from build123d import *

# Parameters (mm, degrees)
F1_DEPTH = 612.95
F3_DEPTH = 127.001


with BuildPart() as f1:
    # F0 (on Front) → F1 (new body)
    with BuildSketch(Plane.XZ):
        with BuildLine():
            Line((-53.95, -63.5), (53.95, -63.5))
            ThreePointArc((53.95, -63.5), (60.70287, -60.70287), (63.5, -53.95))
            Line((63.5, -53.95), (63.5, 53.95))
            ThreePointArc((63.5, 53.95), (60.70287, 60.70287), (53.95, 63.5))
            Line((53.95, 63.5), (-53.95, 63.5))
            ThreePointArc((-53.95, 63.5), (-60.70287, 60.70287), (-63.5, 53.95))
            Line((-63.5, 53.95), (-63.5, -53.95))
            ThreePointArc((-63.5, -53.95), (-60.70287, -60.70287), (-53.95, -63.5))
        make_face()
        with BuildLine():
            ThreePointArc((58.7255, -53.9505), (57.326935, -57.326935), (53.9505, -58.7255))
            Line((53.9505, -58.7255), (-53.9505, -58.7255))
            ThreePointArc((-53.9505, -58.7255), (-57.326935, -57.326935), (-58.7255, -53.9505))
            Line((-58.7255, -53.9505), (-58.7255, 53.9505))
            ThreePointArc((-58.7255, 53.9505), (-57.326935, 57.326935), (-53.9505, 58.7255))
            Line((-53.9505, 58.7255), (53.9505, 58.7255))
            ThreePointArc((53.9505, 58.7255), (57.326935, 57.326935), (58.7255, 53.9505))
            Line((58.7255, 53.9505), (58.7255, -53.9505))
        make_face(mode=Mode.SUBTRACT)
    extrude(amount=F1_DEPTH)

    # F2 (on face) → F3 (cut, through all)
    with BuildSketch(Plane.XY.offset(63.5)):
        with BuildLine():
            Line((-31.75, -142.1), (31.75, -142.1))
            ThreePointArc((31.75, -142.1), (36.240128, -140.240128), (38.1, -135.75))
            Line((38.1, -135.75), (38.1, -110.35))
            ThreePointArc((38.1, -110.35), (36.240128, -105.859872), (31.75, -104))
            Line((31.75, -104), (-31.75, -104))
            ThreePointArc((-31.75, -104), (-36.240128, -105.859872), (-38.1, -110.35))
            Line((-38.1, -110.35), (-38.1, -135.75))
            ThreePointArc((-38.1, -135.75), (-36.240128, -140.240128), (-31.75, -142.1))
        make_face()
    extrude(amount=-F3_DEPTH, mode=Mode.SUBTRACT)


solid = f1.part
Source: CAD feature listing. Evaluate the final solid. Frame: model axes, mm. A direction names the side the tool comes from. Coordinates: 2 decimals unless noted, no trailing zeros. Loops run counter-clockwise (first coordinate to the right, second up) from the corner with the lowest first, then second, coordinate; pieces in that order, holes last. Notation, with made-up numbers: M 14,-33.75 L 37,-33.75 A28 ccw 37,-6.75 Z; hole C -16,-6.5 d8. An arc over 180 degrees is marked long. Answer in a Markdown table with one row per item.
Q1. First-contact query: pin 1 (2.5 mm diameter, centred on y = -123.5, z = 60.5, fed in from -X); pin 2 (4 mm diameter, centred on y = -121.5, z = 62, fed in from +X); pin 3 (4 mm diameter, centred on y = -120.5, z = -60, fed in from -X). Flat tips, straight axial feed; report the tip coordinate or a pass-through.
Answers below:
| item | result |
|---|---|
| pin 1 | stops at x = -61.89 |
| pin 2 | stops at x = 61.34 |
| pin 3 | stops at x = -62.6 |
Q2. Draft query along Z for faces 3 (the flat face through (-1, -302, -63.5)), 4 (the flat face through (1, -302, 63.5)), 5 (the flat face through (58.726, -302, 1)), 6 (the flat face through (-63.5, -302, 1)). Return one class per face: pulls with the +Z half, pulls with the -Z half, needs draft (parallel to the pull), parting line crosses it, or undercut.
Answers below:
| item | result |
|---|---|
| face 3 | pulls with the -Z half |
| face 4 | pulls with the +Z half |
| face 5 | undercut |
| face 6 | needs draft |
Q3. Section A-A on x = -19. Return the cut outline in (y, z), plus the area to 3 significant figures.
Answers below:
| item | result |
|---|---|
| outline | M -612.95,-63.5 L -142.1,-63.5 L -142.1,-58.73 L -612.95,-58.73 Z; M -612.95,58.73 L -142.1,58.73 L -142.1,63.5 L -612.95,63.5 Z; M -104,-63.5 L 0,-63.5 L 0,-58.73 L -104,-58.73 Z; M -104,58.73 L 0,58.73 L 0,63.5 L -104,63.5 Z |
| area | 5,490 mm^2 |
Q4. Ray query, probe 1 along X at (y, z) = (-231.5, 2.5); probe 2 along X at (y, z) = (-299, 55). Return the intervals inside material, ascending. Write a range as from..to.
Answers below:
| item | result |
|---|---|
| probe 1 | x = -63.5..-58.73, 58.73..63.5 |
| probe 2 | x = -63.44..-58.61, 58.61..63.44 |
Q5. Set-up query: faces 1 (the flat face through (63.5, -302, -1)), 2 (the flat face through (1, -302, -58.726)). Return all of +Z, -Z, +X, -X, +Y, -Y with unobstructed straight access to the full face (end or side cutting, diameter ignored); none if empty.
Answers below:
| item | result |
|---|---|
| face 1 | +Z, -Z, +X, +Y, -Y |
| face 2 | +Y, -Y |
Q6. Section B-B on z = -36. Return the cut outline in (x, y).
Answers below:
| item | result |
|---|---|
| outline | M -63.5,-612.95 L -58.73,-612.95 L -58.73,0 L -63.5,0 Z; M 58.73,-612.95 L 63.5,-612.95 L 63.5,0 L 58.73,0 Z |
